Source: CAD feature listing. Evaluate the final solid. Frame: model axes, mm. Face numbers are marked on the shaded views. A direction names the side the tool comes from. Round coordinates to 2 decimals unless told otherwise and drop trailing zeros. Order: outer loops, then holes, each group sorted by start corner. A loop starts at its lowest first (then second) coordinate and runs counter-clockwise, first axis right, second up. Notation, with made-up numbers: M 36.25,76.25 L 53.25,76.25 A28 ccw 53.25,101.25 Z; hole C -10.75,-23 d3. An arc over 180 degrees is marked long. Use one line per item in the form item = value. Start each with the question number.
Q1. Material intervals for probe 1 along X at (y, z) = (0.1, -4.25); probe 2 along Z at (x, y) = (0.75, -1.3); probe 3 along Z at (x, y) = (-0.25, -1.2), sorted ascending.
Q2. Contact query for flat-ended pins moving along their axis: pin 1 (0.8 mm diameter, centred on x = 0, y = -0.5, fed in from +Z); pin 2 (0.6 mm diameter, centred on y = 0.5, z = -2.5, fed in from +X). Output: stop coordinate, or through.
Q3. Reachability of the marked faces 5 and 6 from +Z, -Z, +X, -X, +Y, -Y: full face, straight path, thin tool, end or side. Return the list, or none.
Q4. Section C-C (y = -0.8). Return the cut outline in (x, z), plus the area to 3 significant figures.
Q5. Pull-direction query (X, two-part tool) for the marked faces 1, 2, 3 and 4; classes: pulls with the +X half, pulls with the -X half, needs draft (parallel to the pull), parting line crosses it, or undercut.
from build123d import *

# Parameters (mm, degrees)
SKETCH1_W      = 10
SKETCH1_H      = 20
SKETCH1_W_2    = 2
SKETCH1_H_2    = 12
EXTRUDE1_DEPTH = 1.5
FILLET1_RADIUS = 5
FILLET1_LENGTH = 3
FILLET5_RADIUS = 5
FILLET5_LENGTH = 3
FILLET3_R      = 0.5
FILLET4_R      = 0.5
FILLET6_R      = 1.5


with BuildPart() as part:
    # Sketch1 → Extrude1 (new, symmetric)
    with BuildSketch(Plane(origin=(0, 0, 0), x_dir=(1, 0, 0), z_dir=(0, 1, 0))):
        Rectangle(SKETCH1_W, SKETCH1_H)
        Rectangle(SKETCH1_W_2, SKETCH1_H_2, mode=Mode.SUBTRACT)
    extrude(amount=EXTRUDE1_DEPTH, both=True)

    # Fillet1: full round fillet: the end face becomes a half cylinder, R = half its width
    fillet1_face = Plane((0, 0, 10), x_dir=(0, 1, 0), z_dir=(0, 0, 1))  # on the end face: x along it, z out of the body
    fillet1_slab = fillet1_face.offset(-FILLET1_RADIUS / 2) * Box(FILLET1_LENGTH, 2 * FILLET1_RADIUS, FILLET1_RADIUS, mode=Mode.PRIVATE)  # the body's end, R deep
    fillet1_round = Plane((0, 0, 5), x_dir=(0, 0, 1), z_dir=(0, 1, 0)) * Cylinder(FILLET1_RADIUS, FILLET1_LENGTH, mode=Mode.PRIVATE)  # its axis R under the face
    add(fillet1_slab - fillet1_round, mode=Mode.SUBTRACT)

    # Fillet5: full round fillet: the end face becomes a half cylinder, R = half its width
    fillet5_face = Plane((0, 0, -10), x_dir=(0, 1, 0), z_dir=(0, 0, -1))  # on the end face: x along it, z out of the body
    fillet5_slab = fillet5_face.offset(-FILLET5_RADIUS / 2) * Box(FILLET5_LENGTH, 2 * FILLET5_RADIUS, FILLET5_RADIUS, mode=Mode.PRIVATE)  # the body's end, R deep
    fillet5_round = Plane((0, 0, -5), x_dir=(0, 0, -1), z_dir=(0, 1, 0)) * Cylinder(FILLET5_RADIUS, FILLET5_LENGTH, mode=Mode.PRIVATE)  # its axis R under the face
    add(fillet5_slab - fillet5_round, mode=Mode.SUBTRACT)

    # Fillet3
    fillet3_edges = [part.edges().sort_by_distance(p)[0] for p in [
        (-1, 0, -6),
        (-1, 0, 6),
        (1, 0, 6),
        (1, 0, -6),
    ]]
    fillet(fillet3_edges, radius=FILLET3_R)

    # Fillet4
    fillet4_edges = [part.edges().sort_by_distance(p)[0] for p in [
        (1, -1.5, 0),
        (1, 1.5, 0),
        (0, -1.5, -6),
        (0, 1.5, -6),
        (-1, -1.5, 0),
        (-1, 1.5, 0),
        (0, -1.5, 6),
        (0, 1.5, 6),
        (0.853553391, -1.5, -5.853553391),
        (0.853553391, 1.5, -5.853553391),
        (-0.853553391, -1.5, -5.853553391),
        (-0.853553391, 1.5, -5.853553391),
        (0.853553391, -1.5, 5.853553391),
        (0.853553391, 1.5, 5.853553391),
        (-0.853553391, -1.5, 5.853553391),
        (-0.853553391, 1.5, 5.853553391),
    ]]
    fillet(fillet4_edges, radius=FILLET4_R)

    # Fillet6
    fillet6_edges = [part.edges().sort_by_distance(p)[0] for p in [
        (5, -1.5, 0),
        (5, 1.5, 0),
        (0, 1.5, 10),
        (-5, -1.5, 0),
        (-5, 1.5, 0),
        (0, -1.5, -10),
    ]]
    fillet(fillet6_edges, radius=FILLET6_R - 0.0001)  # a hair under: the kernel refuses the full size


solid = part.part
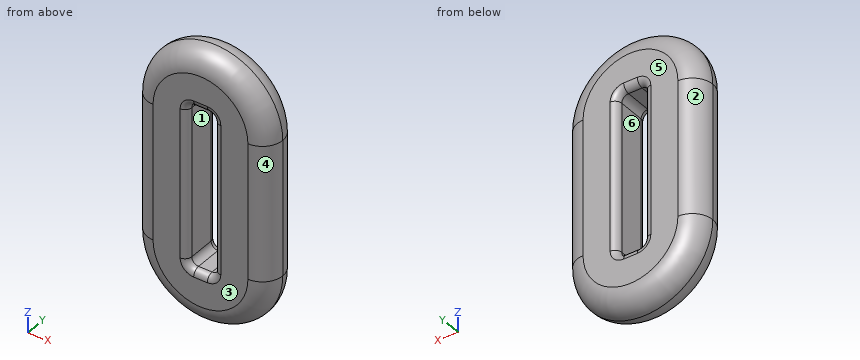
Results list:
q1.probe_1 = -5 to -1, 1 to 5
q1.probe_2 = -9.18 to -6.05, 6.05 to 9.18
q1.probe_3 = -9.39 to -6.04, 6.04 to 9.39
q2.pin_1 = 10
q2.pin_2 = 4.99
q3.face_5 = +Z, -Z, +X, -X, +Y
q3.face_6 = +Y, -Y
q4.outline = M -4.77,-5 A4.77 ccw 4.77,-5 L 4.77,5 A4.77 ccw -4.77,5 Z; hole M -1,-5.5 A0.5 ccw -0.5,-6 L 0.5,-6 A0.5 ccw 1,-5.5 L 1,5.5 A0.5 ccw 0.5,6 L -0.5,6 A0.5 ccw -1,5.5 Z
q4.area = 143 mm2
q5.face_1 = undercut
q5.face_2 = pulls with the -X half
q5.face_3 = needs draft
q5.face_4 = pulls with the +X half
